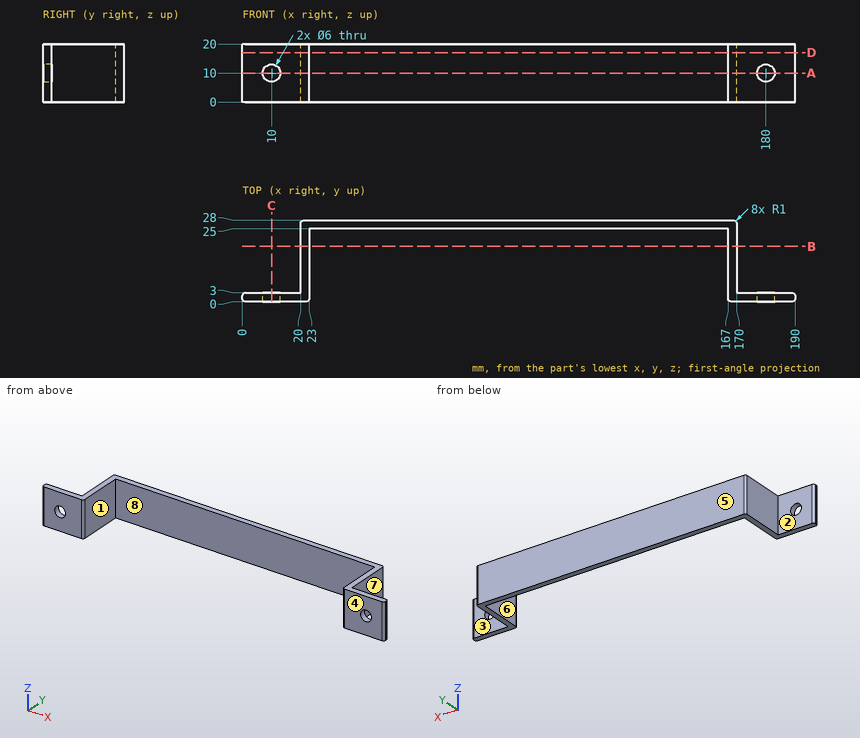
Can you work these out from the drawing? Everything is in mm from the part's minimum corner. A direction names the side the tool comes from. Give positions to 0.01 mm unless a question says otherwise; leave off trailing zeros. Order: outer loops, then holes, each group sorted by start corner. A loop starts at its lowest first (then second) coordinate and runs counter-clockwise, first axis right, second up.
1. I need wall thicknesses on L1, parallel to X at y = 0.95, z = 10; L2, parallel to X at y = 19, z = 10.75; L3, parallel to Z at x = 180, y = 2.15. Which ranges of each line are inside material? Lowest first, please.
2. Suppose I cut it at C-C (x = 10). List the corners of the cut face in (y, z) for me.
3. Suppose I cut it at D-D (z = 17). List the corners of the cut face in (x, y) for me, plus the area to 3 significant figures.
4. For the marked faces 1, 2, 3 and 4, which set-ups out of +Z, -Z, +X, -X, +Y, -Y let a thin tool reach every point of the face, with its end or its side?
5. Will these pins go through, and if not, where does the flat tip stop? P1, Ø6, axis at x = 159.5, z = 14, coming from the -Y side; P2, Ø1, axis at y = 22, z = 6.5, coming from the +X side; P3, Ø6, axis at y = 14, z = 3, coming from the -X side.
6. Suppose I cut it at B-B (y = 19). List the corners of the cut face in (x, z) for me.
7. Suppose I cut it at A-A (z = 10). List the corners of the cut face in (x, y) for me, plus the area to 3 significant figures.
8. We'd pull the mould along X, two halves only. Please class the marked faces 5, 6, 7 and 8: pulls with the +X half, pulls with the -X half, needs draft (parallel to the pull), parting line crosses it, or undercut.
Solved:
1. L1: x = 0 to 7, 13 to 23, 167 to 177, 183 to 190
1. L2: x = 20 to 23, 167 to 170
1. L3: z = 0 to 7, 13 to 20
2. outline: (0, 0) - (3, 0) - (3, 7) - (0, 7) - close; (0, 13) - (3, 13) - (3, 20) - (0, 20) - close
3. outline: (0, 1) arc R1 ccw to (1, 0) - (22, 0) arc R1 ccw to (23, 1) - (23, 25) - (167, 25) - (167, 1) arc R1 ccw to (168, 0) - (189, 0) arc R1 ccw to (190, 1) - (190, 2) arc R1 ccw to (189, 3) - (170, 3) - (170, 27) arc R1 ccw to (169, 28) - (21, 28) arc R1 ccw to (20, 27) - (20, 3) - (1, 3) arc R1 ccw to (0, 2) - close
3. area: 718 mm2
4. face 1: +Z, -Z, -Y
4. face 2: +Z, -Z, -X, +Y
4. face 3: +Z, -Z, +X, +Y
4. face 4: +Z, -Z, +X, -X, -Y
5. P1: stops at y = 25
5. P2: stops at x = 170
5. P3: stops at x = 20
6. outline: (20, 0) - (23, 0) - (23, 20) - (20, 20) - close; (167, 0) - (170, 0) - (170, 20) - (167, 20) - close
7. outline: (0, 1) arc R1 ccw to (1, 0) - (7, 0) - (7, 3) - (1, 3) arc R1 ccw to (0, 2) - close; (13, 0) - (22, 0) arc R1 ccw to (23, 1) - (23, 25) - (167, 25) - (167, 1) arc R1 ccw to (168, 0) - (177, 0) - (177, 3) - (170, 3) - (170, 27) arc R1 ccw to (169, 28) - (21, 28) arc R1 ccw to (20, 27) - (20, 3) - (13, 3) - close; (183, 0) - (189, 0) arc R1 ccw to (190, 1) - (190, 2) arc R1 ccw to (189, 3) - (183, 3) - close
7. area: 682 mm2
8. face 5: needs draft
8. face 6: undercut
8. face 7: pulls with the +X half
8. face 8: undercut
